```python
from build123d import *

# Parameters (mm, degrees)
F1_DEPTH = 2
F2_DEPTH = 15
F4_DEPTH = 4
F5_SIZE  = 1


with BuildPart() as f1:
    # F0 (on Top) → F1 (new body)
    with BuildSketch(Plane.XY):
        with BuildLine():
            Line((-41.924741, 25.953611), (-41.924741, 21.040638))
            ThreePointArc((-41.924741, 21.040638), (-31.332281, -4.229339), (-16.396854, 18.742492))
            Line((-16.396854, 18.742492), (-16.396854, 24.531709))
            Line((-16.396854, 24.531709), (-16.396854, 50.408155))
            Line((-16.396854, 50.408155), (-41.924741, 50.408155))
            Line((-41.924741, 50.408155), (-41.924741, 25.953611))
        make_face()
        with BuildLine():
            ThreePointArc((-16.396854, 18.742492), (-31.332281, -4.229339), (-41.924741, 21.040638))
            Line((-41.924741, 21.040638), (-41.924741, 25.953611))
            ThreePointArc((-41.924741, 25.953611), (-30.999175, -7.762364), (-16.396854, 24.531709))
            Line((-16.396854, 24.531709), (-16.396854, 18.742492))
        make_face()
    extrude(amount=-F1_DEPTH)

    # F0 (on Top) → F2 (join)
    with BuildSketch(Plane.XY):
        with BuildLine():
            ThreePointArc((-16.396854, 18.742492), (-31.332281, -4.229339), (-41.924741, 21.040638))
            Line((-41.924741, 21.040638), (-41.924741, 25.953611))
            ThreePointArc((-41.924741, 25.953611), (-30.999175, -7.762364), (-16.396854, 24.531709))
            Line((-16.396854, 24.531709), (-16.396854, 18.742492))
        make_face()
    extrude(amount=F2_DEPTH)

    # F3 (on Top) → F4 (join)
    with BuildSketch(Plane.XY):
        Polygon((-39.424741, 47.908155), (-39.424741, 50.408155), (-41.924741, 50.408155), (-41.924741, 25.953611), (-41.924741, 21.040638), (-39.424741, 25.953611), align=None)
        Polygon((-16.396854, 24.531709), (-16.396854, 50.408155), (-18.896854, 50.408155), (-18.896854, 47.908155), (-18.896854, 24.531709), (-16.396854, 18.742492), align=None)
    extrude(amount=F4_DEPTH)

    # F5
    f5_edges = [f1.edges().sort_by_distance(p)[0] for p in [
        (-31.332281, -4.229339, 15),
    ]]
    chamfer(f5_edges, length=F5_SIZE)


solid = f1.part
```
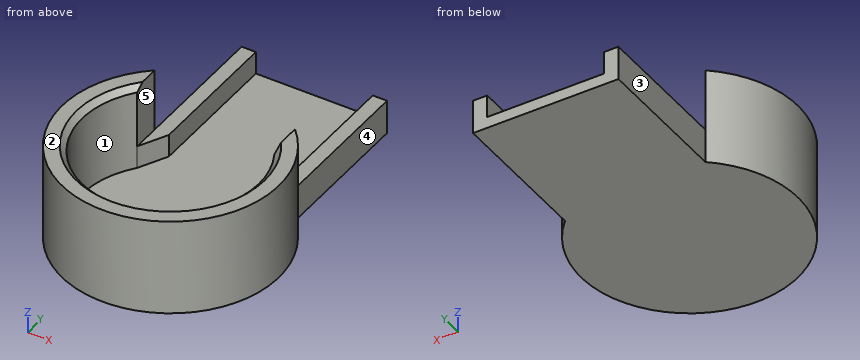
Source: CAD feature listing. Evaluate the final solid. Frame: model axes, mm. Face numbers are marked on the shaded views. A direction names the side the tool comes from. Give positions to 0.01 mm unless a question says otherwise; leave off trailing zeros. Loops run counter-clockwise (first coordinate to the right, second up) from the corner with the lowest first, then second, coordinate; pieces in that order, holes last. Notation, with made-up numbers: M 18,21 L 38,21 A14 ccw 38,42 Z; hole C 69.5,-3.75 d7. An arc over 180 degrees is marked long. Put each result on its own line as item: value.
Q1. Mould query, pull axis X, two halves, no side actions, for the marked faces 3, 4 and 5. Classes: released by +X, released by -X, zero draft, split by the parting line, or undercut.
Response values:
face 3: released by -X
face 4: released by +X
face 5: undercut
Q2. Pin query (flat end, axial travel): P1, Ø4.5, axis at y = 31, z = 1, coming from the -X side; P2, Ø8, axis at y = 5.5, z = 10.5, coming from the +X side; P3, Ø2.5, axis at y = 22.5, z = 11, coming from the +X side. Return the tip coordinate at first contact, or that it passes through.
Response values:
P1: stops at x = -41.92
P2: stops at x = -11.02
P3: stops at x = -13.81
Q3. Section A-A (y = 37). Return the cut outline in (x, z), and give its area (3 significant figures).
Response values:
outline: M -41.92,-2 L -16.4,-2 L -16.4,4 L -18.9,4 L -18.9,0 L -39.42,0 L -39.42,4 L -41.92,4 Z
area: 71.1 mm²
Q4. Section B-B (z = 2). Return the cut outline in (x, y), and give its area (3 significant figures).
Response values:
outline: M -41.92,21.04 L -39.42,25.95 L -39.42,50.41 L -41.92,50.41 L -41.92,25.95 A19 ccw long -16.4,24.53 L -16.4,50.41 L -18.9,50.41 L -18.9,24.53 L -16.4,18.74 A15.5 cw long Z
area: 417 mm²
Q5. Reachability of the marked faces 1 and 2 from +Z, -Z, +X, -X, +Y, -Y: full face, straight path, thin tool, end or side. Return the list, or none.
Response values:
face 1: +Z
face 2: +Z, +X, -X, +Y, -Y
Q6. Section C-C (z = 13). Return the cut outline in (x, y), and give its area (3 significant figures).
Response values:
outline: M -41.92,21.04 L -41.92,25.95 A19 ccw long -16.4,24.53 L -16.4,18.74 A15.5 cw long Z
area: 278 mm²
Q7. Line query: probe 1 along X at (y, z) = (11, 1.5); probe 2 along X at (y, z) = (38.5, 1.5); probe 3 along Z at (x, y) = (-18.5, 41). Output: solid intervals per line, ascending. Write a range as [from, to].
Response values:
probe 1: x = [-48.94, -45.44], [-14.44, -10.94]
probe 2: x = [-41.92, -39.42], [-18.9, -16.4]
probe 3: z = [-2, 4]
Q8. Section D-D (z = -1). Return the cut outline in (x, y).
Response values:
outline: M -41.92,25.95 A19 ccw long -16.4,24.53 L -16.4,50.41 L -41.92,50.41 Z
